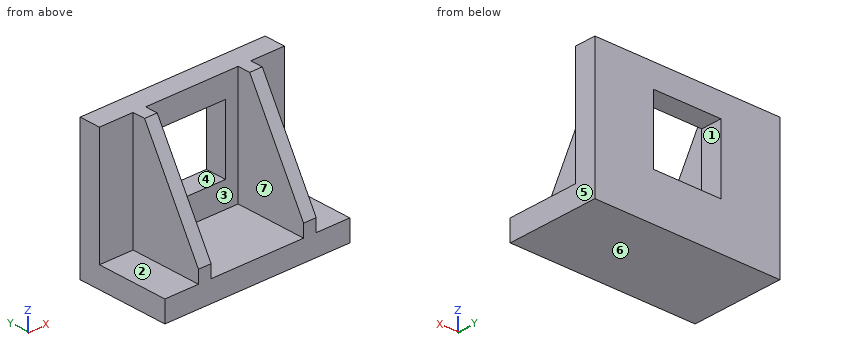
from build123d import *

# Parameters (mm, degrees)
F1_DEPTH = 44
F2_W     = 32
F2_H     = 32
F3_DEPTH = 10.001
F6_DEPTH = 3


# Not quite as in the source:
# - a pattern or mirror of a feature is missing from the dataset's text; its kind, count and spacing are read off the source's solid


with BuildPart() as f1:
    # F0 (on Right) → F1 (new body, symmetric)
    with BuildSketch(Plane.YZ):
        Polygon((0, 10), (0, 0), (44, 0), (44, 65), (34, 65), (34, 10), align=None)
    extrude(amount=F1_DEPTH, both=True)

    # F2 (on face) → F3 (cut, through all)
    with BuildSketch(Plane.XZ.offset(-34)):
        with Locations((0, 38)):
            Rectangle(F2_W, F2_H)
    extrude(amount=-F3_DEPTH, mode=Mode.SUBTRACT)

    # F5 (on offset) → F6 (join, symmetric)
    with BuildSketch(Plane.YZ.offset(25)):
        Polygon((34, 65), (28, 65), (0, 16), (0, 10), (34, 10), align=None)
    f6 = extrude(amount=F6_DEPTH, both=True)

    # F6_copies: F6 across plane
    add(f6.mirror(Plane(origin=(0, 0, 0), x_dir=(0, 0, -1), z_dir=(-1, 0, 0))))


solid = f1.part
Verification items for the finished model (mm, model axes). Face numbers are marked on the shaded views. A direction names the side the tool comes from. Round coordinates to 2 decimals unless told otherwise and drop trailing zeros. Loops run counter-clockwise (first coordinate to the right, second up) from the corner with the lowest first, then second, coordinate; pieces in that order, holes last. Notation, with made-up numbers: (62.5, -3.5) - (67.5, -3.5) arc R31 cw to (67.5, 30.5) - close; hole circle Ø8 at (18.5, 11). An arc over 180 degrees is marked (long way). Answer in a Markdown table with one row per item. Add a question column.
Q1. Gauge pin test, flat ends, axial feed: pin 1 (5 mm diameter, centred on y = 19.5, z = 25, fed in from -X); pin 2 (10 mm diameter, centred on x = -5.5, y = 12.5, fed in from +Z); pin 3 (8 mm diameter, centred on x = 35.5, z = 36.5, fed in from -Y). Record the tip position at first contact, or that the pin passes through.
Q2. Tool access check on the marked faces 1, 2 and 3. Record the directions out of +Z, -Z, +X, -X, +Y, -Y that give a thin tool (end or side, any length) a straight path to the whole face; none if there is none.
Q3. Material ranges on line 1 (Z direction, x = 14.5, y = 42.5); line 2 (X direction, y = 11, z = 17); line 3 (Z direction, x = 33, y = 2.5), recorded low to high.
Q4. Section check A-A on z = 37. Enter the section's corners in (x, y).
Q5. Release check for a two-part mould opening along X. For the marked faces 4, 5, 6 and 7 record: pulls with the +X half, pulls with the -X half, needs draft (parallel to the pull), parting line crosses it, or undercut.
Q6. Section check B-B on y = 35. Enter the section's corners in (x, z), plus the area to 3 significant figures.
Q7. Section check D-D on x = -36. Enter the section's corners in (y, z).
Q8. Section check C-C on x = -5.5. Enter the section's corners in (y, z), plus the area to 3 significant figures.
Found:
| question | item | result |
|---|---|---|
| 1 | pin 1 | stops at x = -28 |
| 1 | pin 2 | stops at z = 10 |
| 1 | pin 3 | stops at y = 34 |
| 2 | face 1 | +Y, -Y |
| 2 | face 2 | +Z, -X, -Y |
| 2 | face 3 | +Z, -Y |
| 3 | line 1 | z = 0 to 22, 54 to 65 |
| 3 | line 2 | x = -28 to -22, 22 to 28 |
| 3 | line 3 | z = 0 to 10 |
| 4 | outline | (-44, 34) - (-28, 34) - (-28, 12) - (-22, 12) - (-22, 34) - (-16, 34) - (-16, 44) - (-44, 44) - close; (16, 34) - (22, 34) - (22, 12) - (28, 12) - (28, 34) - (44, 34) - (44, 44) - (16, 44) - close |
| 5 | face 4 | undercut |
| 5 | face 5 | pulls with the +X half |
| 5 | face 6 | needs draft |
| 5 | face 7 | undercut |
| 6 | outline | (-44, 0) - (44, 0) - (44, 65) - (-44, 65) - close; hole (-16, 22) - (16, 22) - (16, 54) - (-16, 54) - close |
| 6 | area | 4,700 mm² |
| 7 | outline | (0, 0) - (44, 0) - (44, 65) - (34, 65) - (34, 10) - (0, 10) - close |
| 8 | outline | (0, 0) - (44, 0) - (44, 22) - (34, 22) - (34, 10) - (0, 10) - close; (34, 54) - (44, 54) - (44, 65) - (34, 65) - close |
| 8 | area | 670 mm² |
